Verification items for the finished model (mm, model axes). A direction names the side the tool comes from. Give positions to 0.01 mm unless a question says otherwise; leave off trailing zeros. Order: outer loops, then holes, each group sorted by start corner. A loop starts at its lowest first (then second) coordinate and runs counter-clockwise, first axis right, second up.
from build123d import *

# Parameters (mm, degrees)
SKETCH1_W                 = 27.5
SKETCH1_H                 = 57
BOSS_EXTRUDE1_DEPTH       = 25
BOSS_EXTRUDE2_DEPTH       = 2.5
CUT_EXTRUDE1_DEPTH        = 4.5
M4X0_7_TAPPED_HOLE1_D     = 3.3
M4X0_7_TAPPED_HOLE1_DEPTH = 10.1
M4X0_7_TAPPED_HOLE1_TIP   = 0.991420021
CUT_EXTRUDE2_DEPTH        = 8
M4_CLEARANCE_HOLE1_D      = 4.5
F_1_5MM_DOWEL_HOLE1_D     = 1.5
SKETCH11_W                = 15.5
SKETCH11_H                = 42
CUT_EXTRUDE3_DEPTH        = 38.934977264
FILLET1_R                 = 10


with BuildPart() as part:
    # Sketch1 → Boss-Extrude1 (new body)
    with BuildSketch(Plane(origin=(0, 0, 0), x_dir=(1, 0, 0), z_dir=(0, 1, 0))):
        Rectangle(SKETCH1_W, SKETCH1_H)
    extrude(amount=BOSS_EXTRUDE1_DEPTH)

    # Sketch2 → Boss-Extrude2 (add)
    with BuildSketch(Plane.XY.offset(28.5)):
        with BuildLine():
            Line((5.75, 5), (5.75, 25))
            Line((5.75, 25), (11.75, 25))
            Line((11.75, 25), (11.75, 5))
            ThreePointArc((11.75, 5), (8.75, 2), (5.75, 5))
        make_face()
    extrude(amount=BOSS_EXTRUDE2_DEPTH)

    # Sketch3 → Cut-Extrude1 (cut)
    with BuildSketch(Plane(origin=(0, 0, -28.5), x_dir=(-1, 0, 0), z_dir=(0, 0, -1))):
        with BuildLine():
            Line((1.25, 25), (11.25, 25))
            Line((11.25, 25), (11.25, 17.2))
            ThreePointArc((11.25, 17.2), (10.517766953, 15.432233047), (8.75, 14.7))
            Line((8.75, 14.7), (3.75, 14.7))
            ThreePointArc((3.75, 14.7), (1.982233047, 15.432233047), (1.25, 17.2))
            Line((1.25, 17.2), (1.25, 25))
        make_face()
    extrude(amount=-CUT_EXTRUDE1_DEPTH, mode=Mode.SUBTRACT)

    # M4x0.7 Tapped Hole1
    with Locations(Plane.XY.offset(31)):
        with Locations((8.75, 11)):
            Hole(M4X0_7_TAPPED_HOLE1_D / 2, depth=M4X0_7_TAPPED_HOLE1_DEPTH)
            with Locations((0, 0, -(M4X0_7_TAPPED_HOLE1_DEPTH + M4X0_7_TAPPED_HOLE1_TIP / 2))):  # 118° drill point
                Cone(0, M4X0_7_TAPPED_HOLE1_D / 2, M4X0_7_TAPPED_HOLE1_TIP, mode=Mode.SUBTRACT)

    # Sketch6 → Cut-Extrude2 (cut)
    with BuildSketch(Plane(origin=(0, 25, 0), x_dir=(1, 0, 0), z_dir=(0, 1, 0))):
        Polygon((-13.75, 13.5), (1.75, 13.5), (1.75, 28.5), (13.75, 28.5), (13.75, 0), (13.75, -28.5), (11.75, -28.5), (11.75, -31), (5.75, -31), (5.75, -28.5), (-13.75, -28.5), align=None)
    extrude(amount=-CUT_EXTRUDE2_DEPTH, mode=Mode.SUBTRACT)

    # M4 Clearance Hole1 (through all)
    with Locations(Plane.XY.offset(-13.5)):
        with Locations((-6.25, 21.2)):
            Hole(M4_CLEARANCE_HOLE1_D / 2)

    # Ø1.5mm Dowel Hole1 (through all)
    with Locations(Plane(origin=(0, 0, -24), x_dir=(-1, 0, 0), z_dir=(0, 0, -1))):
        with Locations((9.25, 23.2), (3.25, 19.2)):
            Hole(F_1_5MM_DOWEL_HOLE1_D / 2)

    # Sketch11 → Cut-Extrude3 (cut, through all)
    with BuildSketch(Plane(origin=(0, 17, 0), x_dir=(1, 0, 0), z_dir=(0, 1, 0))):
        with Locations((-6, -7.5)):
            Rectangle(SKETCH11_W, SKETCH11_H)
    extrude(amount=-CUT_EXTRUDE3_DEPTH, mode=Mode.SUBTRACT)

    # Fillet1
    fillet1_edges = [part.edges().sort_by_distance(p)[0] for p in [
        (1.75, 8.5, -13.5),
        (13.75, 8.5, -28.5),
    ]]
    fillet(fillet1_edges, radius=FILLET1_R)


solid = part.part
(1) Go/stop test with flat-tipped pins: pin 1 (12 mm diameter, centred on y = 6.5, z = 12, fed in from -X); pin 2 (4 mm diameter, centred on y = 19.5, z = -23, fed in from +X); pin 3 (5.5 mm diameter, centred on x = 8.75, y = 11, fed in from -Z); pin 4 (0.9 mm diameter, centred on x = -3.25, y = 19.2, fed in from +Z). Record where each tip stops, or that it passes through.
Solved:
pin 1: stops at x = 1.75
pin 2: stops at x = 1.75
pin 3: stops at z = -28.24
pin 4: passes through
(2) Section check C-C, the plane z = 2. Enter the section's corners in (x, y).
Solved:
outline: (1.75, 0) - (13.75, 0) - (13.75, 17) - (1.75, 17) - close
(3) Section check B-B, the plane y = 3.5. Enter the section's corners in (x, z).
Solved:
outline: (-13.75, -28.5) - (3.75, -28.5) arc R10 ccw to (13.75, -18.5) - (13.75, 28.5) - (11.35, 28.5) - (11.35, 31) - (6.15, 31) - (6.15, 28.5) - (1.75, 28.5) - (1.75, -3.5) arc R10 cw to (-8.25, -13.5) - (-13.75, -13.5) - close
(4) Set-up check for faces 1 (the cylindrical face through (10.06, 10, 25.88)), 2 (the flat face through (5.75, 11, 30)), 3 (the cylindrical face through (8.8, 2, 29.7)), 4 (the flat face through (-11.25, 21, -26)): record each of +Z, -Z, +X, -X, +Y, -Y from which the full face is reachable in a straight line by a thin tool's end or side.
Solved:
face 1: +Z
face 2: +Z, -X, +Y, -Y
face 3: +Z, -Y
face 4: -Z, +Y
(5) Section check A-A, the plane x = -6.25. Enter the section's corners in (y, z), then the cut area to 3 significant figures.
Solved:
outline: (0, -28.5) - (14.7, -28.5) - (14.7, -24) - (18.95, -24) - (18.95, -13.5) - (17, -13.5) - (17, -13.3) - (0, -13.3) - close; (23.45, -24) - (25, -24) - (25, -13.5) - (23.45, -13.5) - close
area: 285 mm2
(6) Release check for a two-part mould opening along X. For faces 5 (the flat face through (11.75, 11, 30)), 6 (the flat face through (-10, 15, -13.5)), 7 (the flat face through (-6, 14.7, -26)) record: pulls with the +X half, pulls with the -X half, needs draft (parallel to the pull), parting line crosses it, or undercut.
Solved:
face 5: pulls with the +X half
face 6: needs draft
face 7: undercut
(7) Scan lines: line 1 (Y direction, x = -6.25, z = -20.75); line 2 (X direction, y = 11, z = 26.25); line 3 (Y direction, x = -9.25, z = -17.5). Record each from-to range of solid material in increasing order.
Solved:
line 1: y = 0 to 18.95, 23.45 to 25
line 2: x = 1.75 to 7.1, 10.4 to 13.75
line 3: y = 0 to 22.45, 23.95 to 25
(8) Section check D-D, the plane y = 15.75. Enter the section's corners in (x, z), then the cut area to 3 significant figures.
Solved:
outline: (-13.75, -28.5) - (-10.79, -28.5) - (-10.79, -24) - (-1.71, -24) - (-1.71, -28.5) - (3.75, -28.5) arc R10 ccw to (13.75, -18.5) - (13.75, 28.5) - (11.75, 28.5) - (11.75, 31) - (5.75, 31) - (5.75, 28.5) - (1.75, 28.5) - (1.75, -3.5) arc R10 cw to (-8.25, -13.5) - (-13.75, -13.5) - close
area: 891 mm2
